from build123d import *

# Parameters (mm, degrees)
F0_R     = 13
F0_R_2   = 1.525
F0_R_3   = 4.25
F1_DEPTH = 11.1
F2_R     = 5
F2_R_2   = 4.25
F3_DEPTH = 5


with BuildPart() as f1:
    # F0 (on Top) → F1 (new body)
    with BuildSketch(Plane.XY):
        Circle(F0_R)
        with Locations((5.176005, -6.132667)):
            Circle(F0_R_2, mode=Mode.SUBTRACT)
        with Locations((-5.545808, 5.8004)):
            Circle(F0_R_2, mode=Mode.SUBTRACT)
        Circle(F0_R_3, mode=Mode.SUBTRACT)
    extrude(amount=F1_DEPTH)

    # F2 (on face) → F3 (cut)
    with BuildSketch(Plane.XY.offset(11.1)):
        Circle(F2_R)
        Circle(F2_R_2, mode=Mode.SUBTRACT)
    extrude(amount=-F3_DEPTH, mode=Mode.SUBTRACT)


solid = f1.part
Read the model definition and answer for the solid it produces. Units are mm, in the model's axes. A direction names the side the tool comes from. Round coordinates to 2 decimals unless told otherwise and drop trailing zeros. Write each loop counter-clockwise with the first axis right and the second up, starting at its lowest first coordinate (ties: lowest second). Pieces come first, ordered by that corner, then holes. Notation, with made-up numbers: (-10.5, 62.5) - (40.5, 62.5) arc R16 cw to (40.5, 72.5) - close; hole circle Ø6 at (-27, 71). An arc over 180 degrees is marked (long way). One line per question, with ' | ' between items. Start each with the question number.
1. For faces 4 (the face through (-1.08, -4.88, 8.64)), 5 (the face through (2.285, 3.584, 3.007)), determine the directions among +Z, -Z, +X, -X, +Y, -Y from which every point of the face is accessible in a straight line to the end or side of a thin tool.
2. For a pull along X with two mould halves and no side action, classify faces 1 (the face through (-2, -4, 6.1)), 2 (the face through (-10.316, -7.91, 5.472)), 3 (the face through (6, 0, 11.1)) as +X half, -X half, draft (parallel to the pull), parting line (faces both ways), or undercut.
3. Section A-A (x = 0) is taken. Determine the outline of the cut face in (y, z), and give its area (3 significant figures).
4. Section C-C (z = 2.75) is taken. Determine the outline of the cut face in (x, y) (3 decimals).
5. Section D-D (x = 7.5) is taken. Determine the outline of the cut face in (y, z), and give its area (3 significant figures).
6. Each of these flat-tipped pins is pushed along its axis until it touches: pin 1 (3 mm diameter, centred on x = -7.5, z = 8.5, fed in from -Y); pin 2 (3 mm diameter, centred on x = -2.5, y = 0.5, fed in from +Z); pin 3 (4 mm diameter, centred on y = 5.5, z = 8, fed in from +X); pin 4 (2 mm diameter, centred on y = 7.5, z = 6, fed in from +X). Where does it stop, or does it pass through?
7. Find the intervals of material crossed by probe 1 along Y at (x, z) = (-4.5, 8); probe 2 along X at (y, z) = (5.5, 5); probe 3 along X at (y, z) = (1.75, 5), in increasing order. Write a range as [from, to].
Filled in:
1) face 4: +Z | face 5: +Z, -Z
2) face 1: undercut | face 2: parting line | face 3: draft
3) outline: (-13, 0) - (-4.25, 0) - (-4.25, 6.1) - (-5, 6.1) - (-5, 11.1) - (-13, 11.1) - close; (4.25, 0) - (13, 0) - (13, 11.1) - (5, 11.1) - (5, 6.1) - (4.25, 6.1) - close | area: 187 mm²
4) outline: circle Ø26 at (0, 0); hole circle Ø3.05 at (-5.546, 5.8); hole circle Ø8.5 at (0, 0); hole circle Ø3.05 at (5.176, -6.133)
5) outline: (-10.62, 0) - (10.62, 0) - (10.62, 11.1) - (-10.62, 11.1) - close | area: 236 mm²
6) pin 1: y = -11.53 | pin 2: through | pin 3: x = 12.52 | pin 4: x = 11.26
7) probe 1: [-12.2, -2.18], [2.18, 4.69], [6.91, 12.2] | probe 2: [-11.78, -7.04], [-4.05, 11.78] | probe 3: [-12.88, -3.87], [3.87, 12.88]
